Read the model definition and answer for the solid it produces. Units are mm, in the model's axes. Give positions to 0.01 mm unless a question says otherwise; leave off trailing zeros. Order: outer loops, then holes, each group sorted by start corner. A loop starts at its lowest first (then second) coordinate and runs counter-clockwise, first axis right, second up. Notation, with made-up numbers: (79, 82.25) - (87, 82.25) arc R18 cw to (87, 97.25) - close; hole circle Ø3 at (35.25, 60). An arc over 180 degrees is marked (long way). Write each question's results on one line, items separated by ' | '.
from build123d import *

# Parameters (mm, degrees)
SKETCH1_W            = 75
SKETCH1_H            = 75
BOSS_EXTRUDE1_DEPTH  = 3.175
M8_CLEARANCE_HOLE1_D = 9
M5_CLEARANCE_HOLE1_D = 5.5
FILLET1_R            = 10


with BuildPart() as part:
    # Sketch1 → Boss-Extrude1 (new body)
    with BuildSketch(Plane.XY.offset(107.95)):
        with Locations((0, 279.4)):
            Rectangle(SKETCH1_W, SKETCH1_H)
    extrude(amount=BOSS_EXTRUDE1_DEPTH)

    # M8 Clearance Hole1 (through all)
    with Locations(Plane.XY.offset(111.125)):
        with Locations((0, 279.4)):
            Hole(M8_CLEARANCE_HOLE1_D / 2)

    # M5 Clearance Hole1 (through all)
    with Locations(Plane.XY.offset(111.125)):
        with Locations((-27.5, 306.9), (27.5, 306.9), (27.5, 251.9), (-27.5, 251.9)):
            Hole(M5_CLEARANCE_HOLE1_D / 2)

    # Fillet1
    fillet1_edges = [part.edges().sort_by_distance(p)[0] for p in [
        (37.5, 241.9, 109.5375),
        (-37.5, 241.9, 109.5375),
        (-37.5, 316.9, 109.5375),
        (37.5, 316.9, 109.5375),
    ]]
    fillet(fillet1_edges, radius=FILLET1_R)


solid = part.part
(1) Section A-A (x = 0) is taken. Give the vertices of the cut face in (y, z) (3 decimals), plus the area to 3 significant figures.
Conclusion:
outline: (241.9, 107.95) - (274.9, 107.95) - (274.9, 111.125) - (241.9, 111.125) - close; (283.9, 107.95) - (316.9, 107.95) - (316.9, 111.125) - (283.9, 111.125) - close | area: 210 mm^2
(2) This flat-tipped pin is pushed along its axis until it touches: pin 1 (5 mm diameter, centred on x = -27.5, y = 251.9, fed in from -Z). Where does it stop, or does it pass through?
Conclusion:
pin 1: through
(3) Section D-D (z = 109.45) is taken. Give the vertices of the cut face in (x, y).
Conclusion:
outline: (-37.5, 251.9) arc R10 ccw to (-27.5, 241.9) - (27.5, 241.9) arc R10 ccw to (37.5, 251.9) - (37.5, 306.9) arc R10 ccw to (27.5, 316.9) - (-27.5, 316.9) arc R10 ccw to (-37.5, 306.9) - close; hole circle Ø5.5 at (-27.5, 251.9); hole circle Ø5.5 at (-27.5, 306.9); hole circle Ø9 at (0, 279.4); hole circle Ø5.5 at (27.5, 251.9); hole circle Ø5.5 at (27.5, 306.9)
(4) Consider probe 1 along X at (y, z) = (251.9, 109.65); probe 2 along Y at (x, z) = (-27.5, 109); probe 3 along X at (y, z) = (279.4, 109.05). Determine where each line is inside the solid, lowest interval first. Write a range as [from, to].
Conclusion:
probe 1: [-37.5, -30.25], [-24.75, 24.75], [30.25, 37.5] | probe 2: [241.9, 249.15], [254.65, 304.15], [309.65, 316.9] | probe 3: [-37.5, -4.5], [4.5, 37.5]
(5) Section B-B (y = 306) is taken. Give the vertices of the cut face in (x, z) (3 decimals).
Conclusion:
outline: (-37.5, 107.95) - (-30.099, 107.95) - (-30.099, 111.125) - (-37.5, 111.125) - close; (-24.901, 107.95) - (24.901, 107.95) - (24.901, 111.125) - (-24.901, 111.125) - close; (30.099, 107.95) - (37.5, 107.95) - (37.5, 111.125) - (30.099, 111.125) - close
(6) Section C-C (y = 279.4) is taken. Give the vertices of the cut face in (x, z) (3 decimals).
Conclusion:
outline: (-37.5, 107.95) - (-4.5, 107.95) - (-4.5, 111.125) - (-37.5, 111.125) - close; (4.5, 107.95) - (37.5, 107.95) - (37.5, 111.125) - (4.5, 111.125) - close
(7) The mould has two halves that part along X. Classify faces 1 (the face through (-1, 288, 107.95)), 2 (the face through (0.59, 283.86, 109.52)), 3 (the face through (34.49, 314.05, 109.56)), 4 (the face through (-26.904, 249.215, 109.515)): pulls with the +X half, pulls with the -X half, needs draft (parallel to the pull), parting line crosses it, or undercut.
Conclusion:
face 1: needs draft | face 2: undercut | face 3: pulls with the +X half | face 4: undercut
